Autodesk Fusion 360 part; units mm, degrees
sketch "Sketch1" plane through (0, 0, 0) normal (0, 0, 1) x (1, 0, 0)
  line L0 (0, 0) -> (6, 0)
  line L1 (6, 0) -> (6, 15)
  line L2 (6, 15) -> (0, 15)
  line L3 (0, 15) -> (0, 0)
  circle A0 centre (3, 3) radius 1.5
  dimension "d1" = 6
  dimension "d2" = 15
  dimension "d3" = 3
  dimension "d4" = 3
  dimension "d5" = 3
extrude "Extrude1" add sketch "Sketch1" along normal blind 6
sketch "Sketch2" plane through (0, 0, 0) normal (-1, 0, 0) x (0, -1, 0)
  line L0 (-15, 0) -> (0, 0)
  line L1 (0, 0) -> (0, 6)
  line L2 (0, 6) -> (-15, 6)
  line L3 (-15, 6) -> (-15, 0)
  circle A0 centre (-12, 3) radius 1.5
  dimension "d8" = 3
  dimension "d9" = 3
  dimension "d10" = 3
extrude "Extrude2" cut sketch "Sketch2" against normal blind 6 contours A0
The model under review builds one solid part; all positions refer to its coordinate system, in mm. Coordinates: 2 decimals unless noted, no trailing zeros. Loops run counter-clockwise (first coordinate to the right, second up) from the corner with the lowest first, then second, coordinate; pieces in that order, holes last. Notation, with made-up numbers: (89.25, 61.25) -> (139.25, 61.25) arc R30 ccw to (139.25, 89.25) -> close; hole circle Ø4 at (-39, 84). An arc over 180 degrees is marked (long way). Answer as CSV lines item,"result".
Item 1: Take a section at D-D, the plane z = 4.9. State the section outline as (x, y) points, and give its area (3 significant figures).
Results below:
outline,"(0, 0) -> (6, 0) -> (6, 15) -> (0, 15) -> close; hole circle Ø3 at (3, 3)"
area,"82.9 mm2"
Item 2: For L1, parallel to Y at x = 3, z = 2.9; L2, parallel to Y at x = 2.5, z = 3.2; L3, parallel to Y at x = 2.95, z = 0.45, list the stretches that pass through material, from the lowest coordinate up.
Results below:
L1,"y = 0 to 1.5, 4.5 to 10.5, 13.5 to 15"
L2,"y = 0 to 1.59, 4.41 to 10.51, 13.49 to 15"
L3,"y = 0 to 1.5, 4.5 to 15"
Item 3: Draft analysis for pull direction X (two halves, no side actions). For faces 1 (the flat face through (3, 15, 3)), 2 (the flat face through (6, 7, 3)), 3 (the flat face through (0, 8, 3)), 4 (the cylindrical face through (3.806, 1.735, 2.958)), state which applies: +X half, -X half, draft (parallel to the pull), parting line (faces both ways), or undercut.
Results below:
face 1,"draft"
face 2,"+X half"
face 3,"-X half"
face 4,"undercut"
Item 4: Take a section at C-C, the plane y = 3. State the section outline as (x, z) points, and give its area (3 significant figures).
Results below:
outline,"(0, 0) -> (1.5, 0) -> (1.5, 6) -> (0, 6) -> close; (4.5, 0) -> (6, 0) -> (6, 6) -> (4.5, 6) -> close"
area,"18.0 mm2"
Item 5: Take a section at A-A, the plane z = 3. State the section outline as (x, y) points.
Results below:
outline,"(0, 0) -> (6, 0) -> (6, 10.5) -> (0, 10.5) -> close; (0, 13.5) -> (6, 13.5) -> (6, 15) -> (0, 15) -> close; hole circle Ø3 at (3, 3)"
Item 6: Take a section at B-B, the plane x = 3. State the section outline as (y, z) points, and give its area (3 significant figures).
Results below:
outline,"(0, 0) -> (1.5, 0) -> (1.5, 6) -> (0, 6) -> close; (4.5, 0) -> (15, 0) -> (15, 6) -> (4.5, 6) -> close; hole circle Ø3 at (12, 3)"
area,"64.9 mm2"
